from build123d import *

# Parameters (mm, degrees)
SALIENTE_EXTRUIR1_DEPTH = 5
CROQUIS2_R              = 4
CORTAR_EXTRUIR1_DEPTH   = 5


with BuildPart() as part:
    # Croquis1 → Saliente-Extruir1 (new body)
    with BuildSketch(Plane(origin=(0, 0, 0), x_dir=(0, 0, -1), z_dir=(1, 0, 0))):
        Polygon((-17.15051747, 72.789115646), (-17.15051747, 62.789115646), (-12.15051747, 62.789115646), (-12.15051747, 52.789115646), (-17.15051747, 52.789115646), (-17.15051747, 42.789115646), (-12.15051747, 42.789115646), (-12.15051747, 32.789115646), (-17.15051747, 32.789115646), (-17.15051747, 22.789115646), (-12.15051747, 22.789115646), (-12.15051747, 12.789115646), (-17.15051747, 12.789115646), (-17.15051747, 2.789115646), (-12.15051747, 2.789115646), (-12.15051747, -7.210884354), (-17.15051747, -7.210884354), (-17.15051747, -17.210884354), (-12.15051747, -17.210884354), (-12.15051747, -27.210884354), (-17.15051747, -27.210884354), (-17.15051747, -37.210884354), (-12.15051747, -37.210884354), (-12.15051747, -47.210884354), (-17.15051747, -47.210884354), (-17.15051747, -57.210884354), (-12.15051747, -57.210884354), (-12.15051747, -67.210884354), (-5.15051747, -67.210884354), (-5.15051747, -57.210884354), (-0.15051747, -57.210884354), (-0.15051747, -47.210884354), (-5.15051747, -47.210884354), (-5.15051747, -37.210884354), (-0.15051747, -37.210884354), (-0.15051747, -27.210884354), (-5.15051747, -27.210884354), (-5.15051747, -17.210884354), (-0.15051747, -17.210884354), (-0.15051747, -7.210884354), (-5.15051747, -7.210884354), (-5.15051747, 2.789115646), (-0.15051747, 2.789115646), (-0.15051747, 12.789115646), (-5.15051747, 12.789115646), (-5.15051747, 22.789115646), (-0.15051747, 22.789115646), (-0.15051747, 32.789115646), (-5.15051747, 32.789115646), (-5.15051747, 42.789115646), (-0.15051747, 42.789115646), (-0.15051747, 52.789115646), (-5.15051747, 52.789115646), (-5.15051747, 62.789115646), (-0.15051747, 62.789115646), (-0.15051747, 72.789115646), (-5.15051747, 72.789115646), (-5.15051747, 82.789115646), (-0.15051747, 82.789115646), (-0.15051747, 92.789115646), (-17.15051747, 92.789115646), (-17.15051747, 82.789115646), (-12.15051747, 82.789115646), (-12.15051747, 72.789115646), align=None)
    extrude(amount=SALIENTE_EXTRUIR1_DEPTH)

    # Croquis2 → Cortar-Extruir1 (cut)
    with BuildSketch(Plane(origin=(5, 0, 0), x_dir=(0, 0, -1), z_dir=(1, 0, 0))):
        with Locations((-6.65051747, 26.874115646)):
            Circle(CROQUIS2_R)
    extrude(amount=-CORTAR_EXTRUIR1_DEPTH, mode=Mode.SUBTRACT)


solid = part.part
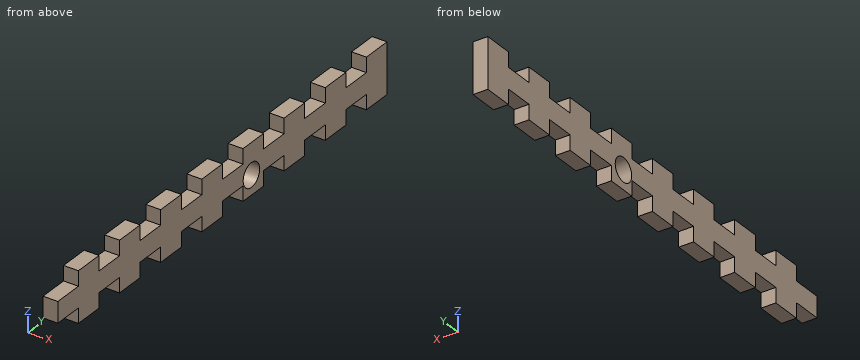
Verification items for the finished model (mm, model axes). Give positions to 0.01 mm unless a question says otherwise; leave off trailing zeros. Write each loop counter-clockwise with the first axis right and the second up, starting at its lowest first coordinate (ties: lowest second). Pieces come first, ordered by that corner, then holes. Notation, with made-up numbers: M 57,14 L 103,14 A29 cw 103,40 Z; hole C 17.25,10.25 d1. An arc over 180 degrees is marked long. Put each result on its own line as item: value. Start each with the question number.
1. Scan lines: line 1 along Y through (x, z) = (3.8, 6.5); line 2 along Y through (x, z) = (2.95, 7.5); line 3 along Z through (x, y) = (3.75, 39.5). Record each from-to range of solid material in increasing order. Write a range as [from, to].
2. Section check C-C (y = 57). Record the cut outline in (x, z), and give its area (3 significant figures).
3. Section check A-A (z = 15.5). Give the number of separate pieces and of enclosed holes in the cut face, and give its area (3 significant figures).
4. Section check B-B (z = 8.75). Record the cut outline in (x, y), and give its area (3 significant figures).
5. Go/stop test with flat-tipped pins: pin 1 Ø1.5 at (x, y) = (2, 40) entering from -Z; pin 2 Ø3 at (x, z) = (3.5, 13.5) entering from -Y; pin 3 Ø2.5 at (x, z) = (1.5, 1.5) entering from -Y; pin 4 Ø2.5 at (x, y) = (3.5, -1) entering from +Z. Record where each tip stops, or that it passes through.
Answer list:
1. line 1: [-67.21, 22.88], [30.87, 92.79]
1. line 2: [-67.21, 22.97], [30.78, 92.79]
1. line 3: [5.15, 12.15]
2. outline: M 0,5.15 L 5,5.15 L 5,12.15 L 0,12.15 Z
2. area: 35.0 mm2
3. separate pieces: 8
3. enclosed holes: 0
3. area: 400 mm2
4. outline: M 0,-67.21 L 5,-67.21 L 5,23.47 L 0,23.47 Z; M 0,30.28 L 5,30.28 L 5,92.79 L 0,92.79 Z
4. area: 766 mm2
5. pin 1: z = 5.15
5. pin 2: y = -67.21
5. pin 3: y = -57.21
5. pin 4: z = 12.15
